Read the model definition and answer for the solid it produces. Units are mm, in the model's axes. Face numbers are marked on the shaded views. A direction names the side the tool comes from. Coordinates: 2 decimals unless noted, no trailing zeros. Loops run counter-clockwise (first coordinate to the right, second up) from the corner with the lowest first, then second, coordinate; pieces in that order, holes last. Notation, with made-up numbers: (4, -9.75) -> (15, -9.75) arc R27 ccw to (15, 8.25) -> close; hole circle Ø9 at (41.5, 66.5). An arc over 180 degrees is marked (long way). Answer in a Markdown table with one row per item.
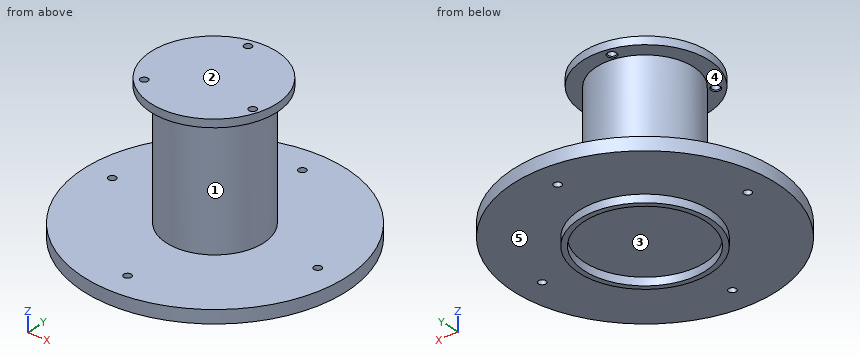
```python
from build123d import *

# Parameters (mm, degrees)
SKETCH_1_R                     = 18.5
EXTRUDE_1_DEPTH                = 50
SKETCH_2_R                     = 50
EXTRUDE_2_DEPTH                = 5
SKETCH_3_R                     = 25
SKETCH_3_R_2                   = 23
EXTRUDE_3_DEPTH                = 3
SKETCH_4_R                     = 1.45
CUT_EXTRUDE_1_DEPTH            = 23
SKETCH_5_R                     = 24
EXTRUDE_4_DEPTH                = 3
HOLE_WIZARD_M3_5_3_D           = 2.9
HOLE_WIZARD_M3_5_3_DEPTH       = 10
HOLE_WIZARD_M3_5_3_CSINK_D     = 3.55
HOLE_WIZARD_M3_5_3_CSINK_ANGLE = 90
HOLE_WIZARD_M3_5_3_TIP         = 0.871247898


with BuildPart() as part:
    # 스케치1 → 보스-돌출1 (new body)
    with BuildSketch(Plane.XY):
        Circle(SKETCH_1_R)
    extrude(amount=EXTRUDE_1_DEPTH)

    # 스케치2 → 보스-돌출2 (add)
    with BuildSketch(Plane(origin=(0, 0, 0), x_dir=(-1, 0, 0), z_dir=(0, 0, -1))):
        Circle(SKETCH_2_R)
    extrude(amount=EXTRUDE_2_DEPTH)

    # 스케치3 → 보스-돌출3 (add)
    with BuildSketch(Plane(origin=(0, 0, -5), x_dir=(-1, 0, 0), z_dir=(0, 0, -1))):
        Circle(SKETCH_3_R)
        Circle(SKETCH_3_R_2, mode=Mode.SUBTRACT)
    extrude(amount=EXTRUDE_3_DEPTH)

    # 스케치4 → 컷-돌출1 (cut)
    with BuildSketch(Plane(origin=(0, 0, -5), x_dir=(-1, 0, 0), z_dir=(0, 0, -1))):
        with Locations((-40, 0)):
            Circle(SKETCH_4_R)
        with Locations((0, 40)):
            Circle(SKETCH_4_R)
        with Locations((40, 0)):
            Circle(SKETCH_4_R)
        with Locations((0, -40)):
            Circle(SKETCH_4_R)
    extrude(amount=-CUT_EXTRUDE_1_DEPTH, mode=Mode.SUBTRACT)

    # 스케치5 → 보스-돌출4 (add)
    with BuildSketch(Plane.XY.offset(50)):
        with Locations((-0.504488898, 0.115254903)):
            Circle(SKETCH_5_R)
    extrude(amount=-EXTRUDE_4_DEPTH)

    # M3.5 나사 구멍3
    with Locations(Plane(origin=(0, 0, 47), x_dir=(-1, 0, 0), z_dir=(0, 0, -1))):
        with Locations((4.588537545, 20.492567511), (15.452815281, -14.220073836), (-20.041352826, -6.272493675)):
            CounterSinkHole(HOLE_WIZARD_M3_5_3_D / 2, HOLE_WIZARD_M3_5_3_CSINK_D / 2, depth=HOLE_WIZARD_M3_5_3_DEPTH, counter_sink_angle=HOLE_WIZARD_M3_5_3_CSINK_ANGLE)
            with Locations((0, 0, -(HOLE_WIZARD_M3_5_3_DEPTH + HOLE_WIZARD_M3_5_3_TIP / 2))):  # 118° drill point
                Cone(0, HOLE_WIZARD_M3_5_3_D / 2, HOLE_WIZARD_M3_5_3_TIP, mode=Mode.SUBTRACT)


solid = part.part
```
1. A cutting plane is placed at D-D on x = 28.5. Give the vertices of the cut face in (y, z), and give its area (3 significant figures).
A:
| item | result |
|---|---|
| outline | (-41.08, -5) -> (41.08, -5) -> (41.08, 0) -> (-41.08, 0) -> close |
| area | 411 mm2 |
2. The mould has two halves that part along Z. Classify the marked faces 1, 2 and 3: pulls with the +Z half, pulls with the -Z half, needs draft (parallel to the pull), parting line crosses it, or undercut.
A:
| item | result |
|---|---|
| face 1 | undercut |
| face 2 | pulls with the +Z half |
| face 3 | pulls with the -Z half |
3. A cutting plane is placed at C-C on y = 14. Give the vertices of the cut face in (x, z), and give its area (3 significant figures).
A:
| item | result |
|---|---|
| outline | (-48, -5) -> (-20.71, -5) -> (-20.71, -8) -> (-18.25, -8) -> (-18.25, -5) -> (18.25, -5) -> (18.25, -8) -> (20.71, -8) -> (20.71, -5) -> (48, -5) -> (48, 0) -> (12.09, 0) -> (12.09, 47) -> (19.07, 47) -> (19.07, 50) -> (-20.08, 50) -> (-20.08, 47) -> (-12.09, 47) -> (-12.09, 0) -> (-48, 0) -> close |
| area | 1,750 mm2 |
4. A cutting plane is placed at A-A on y = -40. Give the vertices of the cut face in (x, z), and give its area (4 significant figures).
A:
| item | result |
|---|---|
| outline | (-30, -5) -> (-1.45, -5) -> (-1.45, 0) -> (-30, 0) -> close; (1.45, -5) -> (30, -5) -> (30, 0) -> (1.45, 0) -> close |
| area | 285.5 mm2 |
5. A tool of negligible diameter and unlimited length cuts with its end or side. For the marked faces 4 and 5, from which of +Z, -Z, +X, -X, +Y, -Y can it reach the whole face along a straight path? Write none if from no direction.
A:
| item | result |
|---|---|
| face 4 | none |
| face 5 | -Z |
6. Given pin 1 Ø6 at (y, z) = (-5.5, 41.5) entering from +X; pin 2 Ø1.5 at (x, y) = (-1.5, -19.5) entering from -Z; pin 3 Ø8 at (x, y) = (-8, 39.5) entering from +Z, each flat-ended and moving along its own axis, determine where each tip first touches the part or whether it passes through.
A:
| item | result |
|---|---|
| pin 1 | stops at x = 18.33 |
| pin 2 | stops at z = -5 |
| pin 3 | stops at z = 0 |
7. Find the intervals of material crossed by probe 1 along Z at (x, y) = (-10.5, -7.5); probe 2 along Z at (x, y) = (-21.5, -28.5); probe 3 along X at (y, z) = (-1, 19), in increasing order.
A:
| item | result |
|---|---|
| probe 1 | z = -5 to 50 |
| probe 2 | z = -5 to 0 |
| probe 3 | x = -18.47 to 18.47 |
8. A cutting plane is placed at B-B on z = 36. Give the vertices of the cut face in (x, y).
A:
| item | result |
|---|---|
| outline | circle Ø37 at (0, 0) |
